Drawing for the job (mm, zero at the part's lowest x, y, z). Give positions to 0.01 mm unless a question says otherwise; leave off trailing zeros. Answer in a Markdown table with one row per item. Add a question column.
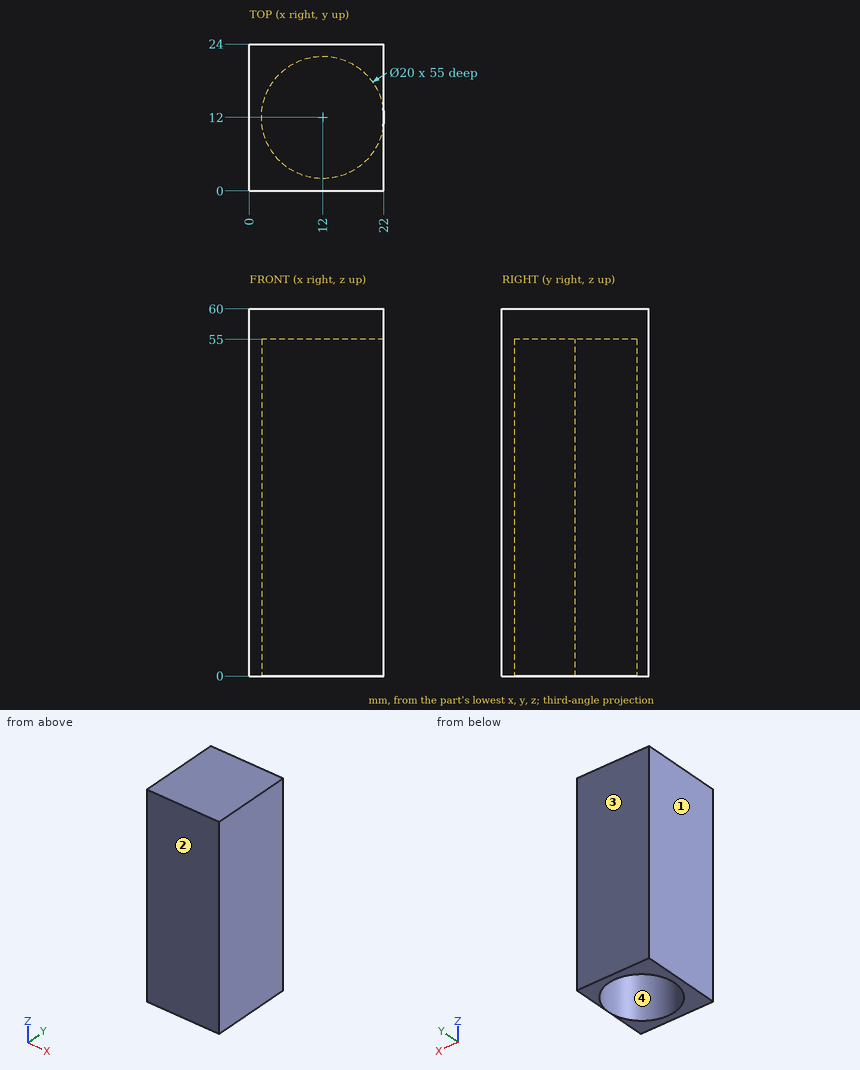
(1) Wall check: line 1 (Y direction, x = 12, z = 23.5); line 2 (Z direction, x = 10.25, y = 16.25); line 3 (Y direction, x = 21, z = 44). Give the ranges that are in metal, low to high.
(2) Pull direction Y, two halves, no side cores. Call the marked faces 1, 2, 3 and 4: +Y half, -Y half, draft (parallel to the pull), parting line (faces both ways), or undercut.
(3) Pin check, flat tip, straight feed: pin 1 (6 mm diameter, centred on x = 11, y = 16, fed in from -Z). Stop position of the tip, or through.
Solution:
| question | item | result |
|---|---|---|
| 1 | line 1 | 0 to 2, 22 to 24 |
| 1 | line 2 | 55 to 60 |
| 1 | line 3 | 0 to 7.64, 16.36 to 24 |
| 2 | face 1 | draft |
| 2 | face 2 | -Y half |
| 2 | face 3 | +Y half |
| 2 | face 4 | undercut |
| 3 | pin 1 | z = 55 |
